from build123d import *

# Parameters (mm, degrees)
BOSS_EXTRUDE1_DEPTH = 16
SKETCH2_W           = 438.581
SKETCH2_H           = 128
SKETCH2_W_2         = 430.581
SKETCH2_H_2         = 110
BOSS_EXTRUDE2_DEPTH = 3
SKETCH3_W           = 440.5822769
SKETCH3_H           = 124
CUT_EXTRUDE1_DEPTH  = 2
SKETCH4_R           = 1.05
CUT_EXTRUDE2_DEPTH  = 2.5
SKETCH5_W           = 30
SKETCH5_H           = 5
CUT_EXTRUDE3_DEPTH  = 6
CUT_EXTRUDE4_DEPTH  = 4
CHAMFER8_SIZE       = 1


with BuildPart() as part:
    # Sketch1 → Boss-Extrude1 (new body)
    with BuildSketch(Plane.XY):
        with BuildLine():
            ThreePointArc((-7, -2), (-5.535533906, -5.535533906), (-2, -7))
            Line((-2, -7), (436.581, -7))
            ThreePointArc((436.581, -7), (440.116533906, -5.535533906), (441.581, -2))
            Line((441.581, -2), (441.581, 116))
            ThreePointArc((441.581, 116), (440.116533906, 119.535533906), (436.581, 121))
            Line((436.581, 121), (-2, 121))
            ThreePointArc((-2, 121), (-5.535533906, 119.535533906), (-7, 116))
            Line((-7, 116), (-7, -2))
        make_face()
        with BuildLine():
            Line((251.291, 114), (306.936, 114))
            Line((306.936, 114), (306.936, 117))
            ThreePointArc((306.936, 117), (307.521786438, 118.414213562), (308.936, 119))
            Line((308.936, 119), (372.936, 119))
            ThreePointArc((372.936, 119), (374.350213562, 118.414213562), (374.936, 117))
            Line((374.936, 117), (374.936, 114))
            Line((374.936, 114), (434.581, 114))
            Line((434.581, 114), (434.581, 0))
            Line((434.581, 0), (374.936, 0))
            Line((374.936, 0), (374.936, -3))
            ThreePointArc((374.936, -3), (374.350213562, -4.414213562), (372.936, -5))
            Line((372.936, -5), (308.936, -5))
            ThreePointArc((308.936, -5), (307.521786438, -4.414213562), (306.936, -3))
            Line((306.936, -3), (306.936, 0))
            Line((306.936, 0), (251.291, 0))
            Line((251.291, 0), (251.291, -3))
            ThreePointArc((251.291, -3), (250.705213562, -4.414213562), (249.291, -5))
            Line((249.291, -5), (185.291, -5))
            ThreePointArc((185.291, -5), (183.876786438, -4.414213562), (183.291, -3))
            Line((183.291, -3), (183.291, 0))
            Line((183.291, 0), (127.646, 0))
            Line((127.646, 0), (127.646, -3))
            ThreePointArc((127.646, -3), (127.060213562, -4.414213562), (125.646, -5))
            Line((125.646, -5), (61.646, -5))
            ThreePointArc((61.646, -5), (60.231786438, -4.414213562), (59.646, -3))
            Line((59.646, -3), (59.646, 0))
            Line((59.646, 0), (0, 0))
            Line((0, 0), (0, 114))
            Line((0, 114), (59.646, 114))
            Line((59.646, 114), (59.646, 117))
            ThreePointArc((59.646, 117), (60.231786438, 118.414213562), (61.646, 119))
            Line((61.646, 119), (125.646, 119))
            ThreePointArc((125.646, 119), (127.060213562, 118.414213562), (127.646, 117))
            Line((127.646, 117), (127.646, 114))
            Line((127.646, 114), (183.291, 114))
            Line((183.291, 114), (183.291, 117))
            ThreePointArc((183.291, 117), (183.876786438, 118.414213562), (185.291, 119))
            Line((185.291, 119), (249.291, 119))
            ThreePointArc((249.291, 119), (250.705213562, 118.414213562), (251.291, 117))
            Line((251.291, 117), (251.291, 114))
        make_face(mode=Mode.SUBTRACT)
    extrude(amount=BOSS_EXTRUDE1_DEPTH)

    # Sketch2 → Boss-Extrude2 (add)
    with BuildSketch(Plane.XY.offset(16)):
        with Locations((217.2905, 57)):
            Rectangle(SKETCH2_W, SKETCH2_H)
        with Locations((217.2905, 57)):
            Rectangle(SKETCH2_W_2, SKETCH2_H_2, mode=Mode.SUBTRACT)
    extrude(amount=-BOSS_EXTRUDE2_DEPTH)

    # Sketch3 → Cut-Extrude1 (cut)
    with BuildSketch(Plane(origin=(0, 0, 0), x_dir=(-1, 0, 0), z_dir=(0, 0, -1))):
        with Locations((-217.28986155, 57)):
            Rectangle(SKETCH3_W, SKETCH3_H)
    extrude(amount=-CUT_EXTRUDE1_DEPTH, mode=Mode.SUBTRACT)

    # Sketch4 → Cut-Extrude2 (cut)
    with BuildSketch(Plane(origin=(0, 0, 2), x_dir=(-1, 0, 0), z_dir=(0, 0, -1))):
        with Locations((-279.1135, 116.5)):
            Circle(SKETCH4_R)
        with Locations((-155.4685, 116.5)):
            Circle(SKETCH4_R)
        with Locations((-279.1135, -2.5)):
            Circle(SKETCH4_R)
        with Locations((-155.4685, -2.5)):
            Circle(SKETCH4_R)
        with Locations((-2, -2.5)):
            Circle(SKETCH4_R)
        with Locations((-2, 116.5)):
            Circle(SKETCH4_R)
        with Locations((-432.581, 116.5)):
            Circle(SKETCH4_R)
        with Locations((-432.581, -2.5)):
            Circle(SKETCH4_R)
    extrude(amount=-CUT_EXTRUDE2_DEPTH, mode=Mode.SUBTRACT)

    # Sketch5 → Cut-Extrude3 (cut)
    with BuildSketch(Plane(origin=(0, 0, 2), x_dir=(-1, 0, 0), z_dir=(0, 0, -1))):
        with Locations((-32, 116.5)):
            Rectangle(SKETCH5_W, SKETCH5_H)
    extrude(amount=-CUT_EXTRUDE3_DEPTH, mode=Mode.SUBTRACT)

    # Sketch6 → Cut-Extrude4 (cut)
    with BuildSketch(Plane.XZ.offset(-119)):
        with BuildLine():
            Line((34.677255015, 2), (27.677255015, 2))
            ThreePointArc((27.677255015, 2), (26.616594843, 2.439339828), (26.177255015, 3.5))
            Line((26.177255015, 3.5), (26.177255015, 4.5))
            ThreePointArc((26.177255015, 4.5), (26.616594843, 5.560660172), (27.677255015, 6))
            Line((27.677255015, 6), (34.677255015, 6))
            ThreePointArc((34.677255015, 6), (35.737915187, 5.560660172), (36.177255015, 4.5))
            Line((36.177255015, 4.5), (36.177255015, 3.5))
            ThreePointArc((36.177255015, 3.5), (35.737915187, 2.439339828), (34.677255015, 2))
        make_face()
    extrude(amount=-CUT_EXTRUDE4_DEPTH, mode=Mode.SUBTRACT)

    # Chamfer8
    chamfer8_edges = [part.edges().sort_by_distance(p)[0] for p in [
        (31.177255015, 121, 6),
        (26.616594843, 121, 5.560660172),
        (26.177255015, 121, 4),
        (26.616594843, 121, 2.439339828),
        (31.177255015, 121, 2),
        (35.737915187, 121, 2.439339828),
        (36.177255015, 121, 4),
        (35.737915187, 121, 5.560660172),
    ]]
    chamfer(chamfer8_edges, length=CHAMFER8_SIZE)


solid = part.part
Model file for the job. Use its own axes, mm. A direction names the side the tool comes from. Give positions to 0.01 mm unless a question says otherwise; leave off trailing zeros. Order: outer loops, then holes, each group sorted by start corner. A loop starts at its lowest first (then second) coordinate and runs counter-clockwise, first axis right, second up. Notation, with made-up numbers: (-7, 53) - (43, 53) arc R21 cw to (43, 87) - close; hole circle Ø4 at (32.25, -23). An arc over 180 degrees is marked (long way). Return JSON: item names as keys, results as strings.
1) Probe line 1 (Y direction, x = 2, z = 3.65); line 2 (Y direction, x = 224.5, z = 10.75); line 3 (X direction, y = 98.5, z = 3.25). List the from-to ranges inside material, lowest first. Write a range as from..to.
Geometry says:
{"line 1": "-7..-3.55, -1.45..0, 114..115.45, 117.55..121", "line 2": "-7..-5, 119..121", "line 3": "-7..0, 434.58..441.58"}
2) Cut at A-A, the plane x = 224.5. Give the cut face in (y, z).
Geometry says:
{"outline": "(-7, 0) - (-5, 0) - (-5, 13) - (2, 13) - (2, 16) - (-7, 16) - close; (112, 13) - (119, 13) - (119, 0) - (121, 0) - (121, 16) - (112, 16) - close"}
3) Pull direction Y, two halves, no side cores. Call faces 3 (the flat face through (220, 121, 8)), 4 (the flat face through (-7, 58, 8)), 5 (the flat face through (30, 0, 7)), 6 (the flat face through (214, -7, 8)): pulls with the +Y half, pulls with the -Y half, needs draft (parallel to the pull), parting line crosses it, or undercut.
Geometry says:
{"face 3": "pulls with the +Y half", "face 4": "needs draft", "face 5": "undercut", "face 6": "pulls with the -Y half"}
4) Cut at B-B, the plane y = 88. Give the cut face in (x, z), plus the area to 3 significant figures.
Geometry says:
{"outline": "(-7, 0) - (-3, 0) - (-3, 2) - (0, 2) - (0, 13) - (2, 13) - (2, 16) - (-7, 16) - close; (432.58, 13) - (434.58, 13) - (434.58, 2) - (437.58, 2) - (437.58, 0) - (441.58, 0) - (441.58, 16) - (432.58, 16) - close", "area": "224 mm²"}
5) Cut at C-C, the plane x = 273.5. Give the cut face in (y, z), plus the area to 3 significant figures.
Geometry says:
{"outline": "(-7, 0) - (-5, 0) - (-5, 2) - (0, 2) - (0, 13) - (2, 13) - (2, 16) - (-7, 16) - close; (112, 13) - (114, 13) - (114, 2) - (119, 2) - (119, 0) - (121, 0) - (121, 16) - (112, 16) - close", "area": "216 mm²"}
6) Flat gauge pins, fed straight in: P1, Ø2.5, axis at x = 432.581, y = 116.5, coming from the -Z side; P2, Ø1.1, axis at y = 119.5, z = 4, coming from the +X side; P3, Ø1.5, axis at y = 117.5, z = 5, coming from the -X side. Where does each tip first touch, or does it go through?
Geometry says:
{"P1": "z = 2", "P2": "x = 440.62", "P3": "x = -6.94"}
7) 3-axis set-ups, long thin cutter, end or side, ignore diameter. For faces 1 (the flat face through (441.581, 56, 8)), 2 (the flat face through (-2, 39, 2)): which of +Z, -Z, +X, -X, +Y, -Y reach the whole face in a straight line?
Geometry says:
{"face 1": "+Z, -Z, +X, +Y, -Y", "face 2": "-Z"}
